```python
from build123d import *

# Parameters (mm, degrees)
BOSS_EXTRUDE3_DEPTH = 7
BOSS_EXTRUDE4_DEPTH = 7
FILLET2_R           = 10
SHELL8_START        = -4
SHELL8_DEPTH        = 8
SHELL8_START_2      = -5
SHELL8_2_OUTLINE_W  = 1
SHELL8_2_OUTLINE_H  = 99
SHELL8_2_DEPTH      = 10
SHELL8_3_DEPTH      = 1
SKETCH14_W          = 8
SKETCH14_H          = 185.360533748
BOSS_EXTRUDE5_DEPTH = 4
FILLET5_R           = 18.82495


with BuildPart() as part:
    # Sketch10 → Boss-Extrude3 (new body)
    with BuildSketch(Plane(origin=(0, 0, 0), x_dir=(1, 0, 0), z_dir=(0, 1, 0))):
        with BuildLine():
            Line((-5, -52.5), (5, -52.5))
            ThreePointArc((5, -52.5), (12.071067812, -49.571067812), (15, -42.5))
            Line((15, -42.5), (15, 42.5))
            ThreePointArc((15, 42.5), (12.071067812, 49.571067812), (5, 52.5))
            Line((5, 52.5), (-5, 52.5))
            ThreePointArc((-5, 52.5), (-12.071067812, 49.571067812), (-15, 42.5))
            Line((-15, 42.5), (-15, -42.5))
            ThreePointArc((-15, -42.5), (-12.071067812, -49.571067812), (-5, -52.5))
        make_face()
    extrude(amount=-BOSS_EXTRUDE3_DEPTH)

    # Sketch11 → Boss-Extrude4 (add, symmetric)
    with BuildSketch(Plane(origin=(0, 0, 0), x_dir=(0, 0, -1), z_dir=(1, 0, 0))):
        Polygon((-71, -133), (-69.505577442, -127.769521047), (-90.305891411, -127.769521047), (-95.800313969, -147), (-75, -147), align=None)
        Polygon((0, -133), (-50.199686031, -133), (-71, -133), (-75, -147), (0, -147), align=None)
        Polygon((50.199686031, -133), (0, -133), (0, -147), (75, -147), (71, -133), align=None)
        Polygon((-14.199686031, -7), (-35, -7), (-69.505577442, -127.769521047), (-71, -133), (-50.199686031, -133), align=None)
        Polygon((35, -7), (14.199686031, -7), (50.199686031, -133), (71, -133), (69.505577442, -127.769521047), align=None)
        Polygon((90.305891411, -127.769521047), (69.505577442, -127.769521047), (71, -133), (75, -147), (95.800313969, -147), align=None)
    extrude(amount=BOSS_EXTRUDE4_DEPTH, both=True)

    # Fillet2
    fillet2_edges = [part.edges().sort_by_distance(p)[0] for p in [
        (0, -133, -50.199686031),
        (0, -133, 50.199686031),
        (0, -127.769521047, 69.505577442),
        (0, -127.769521047, 90.305891411),
        (0, -127.769521047, -90.305891411),
        (0, -127.769521047, -69.505577442),
    ]]
    fillet(fillet2_edges, radius=FILLET2_R)

    # Shell8: read off the stored shape, not the designer's step
    # Shell8 outline → Shell8 (cut)
    with BuildSketch(Plane.YZ.offset(SHELL8_START)):
        with BuildLine():
            Line((-3, -49.5), (-3, 49.5))
            Line((-3, 49.5), (-4, 49.5))
            Line((-4, 49.5), (-4, 31.022810047))
            Line((-4, 31.022810047), (-121.34089571, 64.54878025))
            ThreePointArc((-121.34089571, 64.54878025), (-128.148053473, 69.220049899), (-130.769521047, 77.04859157))
            Line((-130.769521047, 77.04859157), (-130.769521047, 82.762877284))
            ThreePointArc((-130.769521047, 82.762877284), (-132.18108051, 86.978245876), (-135.846473152, 89.493544917))
            Line((-135.846473152, 89.493544917), (-147, 92.680266874))
            Line((-147, 92.680266874), (-147, -92.680266874))
            Line((-147, -92.680266874), (-135.846473152, -89.493544917))
            ThreePointArc((-135.846473152, -89.493544917), (-132.18108051, -86.978245876), (-130.769521047, -82.762877284))
            Line((-130.769521047, -82.762877284), (-130.769521047, -77.04859157))
            ThreePointArc((-130.769521047, -77.04859157), (-128.148053473, -69.220049899), (-121.34089571, -64.54878025))
            Line((-121.34089571, -64.54878025), (-4, -31.022810047))
            Line((-4, -31.022810047), (-4, -49.5))
            Line((-4, -49.5), (-3, -49.5))
        make_face()
        with BuildLine():
            Line((-4, 16.462590269), (-4, -16.462590269))
            Line((-4, -16.462590269), (-119.428625337, -49.442197508))
            ThreePointArc((-119.428625337, -49.442197508), (-130.828541671, -47.320918614), (-136, -36.942386189))
            Line((-136, -36.942386189), (-136, 36.942386189))
            ThreePointArc((-136, 36.942386189), (-130.828541671, 47.320918614), (-119.428625337, 49.442197508))
            Line((-119.428625337, 49.442197508), (-4, 16.462590269))
        make_face(mode=Mode.SUBTRACT)
    extrude(amount=SHELL8_DEPTH, mode=Mode.SUBTRACT)

    # Shell8 2 outline → Shell8 2 (cut)
    with BuildSketch(Plane.YZ.offset(SHELL8_START_2)):
        with Locations((-3.5, 0)):
            Rectangle(SHELL8_2_OUTLINE_W, SHELL8_2_OUTLINE_H)
    extrude(amount=SHELL8_2_DEPTH, mode=Mode.SUBTRACT)

    # Shell8 3 outline → Shell8 3 (cut)
    with BuildSketch(Plane(origin=(0, 0, 0), x_dir=(1, 0, 0), z_dir=(0, 1, 0)).offset(SHELL8_START)):
        with BuildLine():
            Line((5, 49.5), (5, -49.5))
            ThreePointArc((5, -49.5), (9.949747468, -47.449747468), (12, -42.5))
            Line((12, -42.5), (12, 42.5))
            ThreePointArc((12, 42.5), (9.949747468, 47.449747468), (5, 49.5))
        make_face()
        with BuildLine():
            Line((-12, 42.5), (-12, -42.5))
            ThreePointArc((-12, -42.5), (-9.949747468, -47.449747468), (-5, -49.5))
            Line((-5, -49.5), (-5, 49.5))
            ThreePointArc((-5, 49.5), (-9.949747468, 47.449747468), (-12, 42.5))
        make_face()
    extrude(amount=SHELL8_3_DEPTH, mode=Mode.SUBTRACT)

    # Sketch14 → Boss-Extrude5 (add)
    with BuildSketch(Plane.XZ.offset(147)):
        Rectangle(SKETCH14_W, SKETCH14_H)
    extrude(amount=-BOSS_EXTRUDE5_DEPTH)

    # Fillet5
    fillet5_edges = [part.edges().sort_by_distance(p)[0] for p in [
        (0, -7, 14.199686031),
        (0, -7, -14.199686031),
    ]]
    fillet(fillet5_edges, radius=FILLET5_R - 0.0001)  # a hair under: the kernel refuses the full size


solid = part.part
```
CAD build for the part. Positions are in the model's coordinates, mm. A direction names the side the tool comes from. Round coordinates to 2 decimals unless told otherwise and drop trailing zeros. Write each loop counter-clockwise with the first axis right and the second up, starting at its lowest first coordinate (ties: lowest second). Pieces come first, ordered by that corner, then holes. Notation, with made-up numbers: (42, -27) - (97, -27) arc R10 cw to (97, -8) - close; hole circle Ø2 at (-8, 21). An arc over 180 degrees is marked (long way). Return JSON: item names as keys, results as strings. Group by question number.
Item 1: Flat gauge pins, fed straight in: pin 1 Ø4.5 at (x, z) = (1.5, 79) entering from +Y; pin 2 Ø12 at (y, z) = (-36.5, 41) entering from +X; pin 3 Ø6 at (y, z) = (-128.5, 22) entering from +X; pin 4 Ø3.5 at (x, y) = (0.5, -4) entering from +Z. Where does each tip first touch, or does it go through?
Item 2: Band-saw the part on B-B on y = -14.5. List the corners of the cut face in (x, z).
Item 3: 3-axis set-ups, long thin cutter, end or side, ignore diameter. For faces 1 (the face through (7, -134, 0)), 2 (the face through (-0.056, -130.694, -47.421)), 3 (the face through (-0.098, -10.694, 11.2)): which of +Z, -Z, +X, -X, +Y, -Y reach the whole face in a straight line?
Item 4: Mould opens along Y. For faces 4 (the face through (12.15, -3.45, -49.49)), 5 (the face through (10, -3.5, -47.4)), 6 (the face through (0, 0, -1)) say: +Y half, -Y half, draft (parallel to the pull), parting line (faces both ways), or undercut.
Item 5: Probe probe 1 along X at (y, z) = (-41, 30); probe 2 along Y at (x, z) = (-0.5, -9.5); probe 3 along Z at (x, y) = (1, -13.5). List the from-to ranges inside material, lowest first.
Item 6: Band-saw the part on D-D on z = -62. List the corners of the cut face in (x, y).
Item 7: Band-saw the part on A-A on z = -10. List the corners of the cut face in (x, y), plus the area to 3 significant figures.
Item 8: Band-saw the part on C-C on x = 10. List the corners of the cut face in (y, z).
Resolved:
{
 "1": {"pin 1": "stops at y = -127.77", "pin 2": "stops at x = 7", "pin 3": "passes through", "pin 4": "stops at z = 52.5"},
 "2": {"outline": "(-7, -37.14) - (7, -37.14) - (7, -15.04) - (-7, -15.04) - close; (-7, 15.04) - (7, 15.04) - (7, 37.14) - (-7, 37.14) - close; hole (-4, -34.02) - (4, -34.02) - (4, -19.46) - (-4, -19.46) - close; hole (-4, 19.46) - (4, 19.46) - (4, 34.02) - (-4, 34.02) - close"},
 "3": {"face 1": "+Z, -Z, +X, -Y", "face 2": "none", "face 3": "+X, -X"},
 "4": {"face 4": "draft", "face 5": "undercut", "face 6": "+Y half"},
 "5": {"probe 1": "x = -7 to -4, 4 to 7", "probe 2": "y = -147 to -143, -136 to -133, -9.57 to -4, -3 to 0", "probe 3": "z = -36.86 to -33.74, -19.18 to -14.23, 14.23 to 19.18, 33.74 to 36.86"},
 "6": {"outline": "(-7, -147) - (7, -147) - (7, -101.5) - (-7, -101.5) - close; hole (-4, -143) - (4, -143) - (4, -112.42) - (-4, -112.42) - close"},
 "7": {"outline": "(-15, -7) - (-7, -7) - (-7, -9.88) - (7, -9.88) - (7, -7) - (15, -7) - (15, 0) - (-15, 0) - close; (-7, -147) - (7, -147) - (7, -133) - (-7, -133) - close; hole (-12, -4) - (12, -4) - (12, -3) - (-12, -3) - close; hole (-4, -143) - (4, -143) - (4, -136) - (-4, -136) - close", "area": "366 mm²"},
 "8": {"outline": "(-7, -51.16) - (0, -51.16) - (0, 51.16) - (-7, 51.16) - close; hole (-4, -47.4) - (-3, -47.4) - (-3, 47.4) - (-4, 47.4) - close"}
}
